```python
from build123d import *

# Parameters (mm, degrees)
SKETCH008_W  = 20
SKETCH008_H  = 20
PAD004_DEPTH = 3
PAD005_DEPTH = 3
SKETCH014_W  = 3
SKETCH014_H  = 3
PAD010_DEPTH = 1.5
SKETCH015_W  = 3
SKETCH015_H  = 3
PAD011_DEPTH = 1.5


with BuildPart() as part:
    # Sketch008 → Pad004 (new body)
    with BuildSketch(Plane.XZ):
        with BuildLine():
            Line((-68, -38.5), (3, -38.5))
            Line((3, -3), (3, -38.5))
            Line((0, -3), (3, -3))
            ThreePointArc((0, 3), (-6.5, 0), (0, -3))
            Line((0, 3), (3, 3))
            Line((3, 3), (3, 38.5))
            Line((3, 38.5), (-68, 38.5))
            Line((-68, 38.5), (-68, -38.5))
        make_face()
        with BuildLine():
            ThreePointArc((-12.5, 15), (-15, 17.5), (-17.5, 15))
            Line((-17.5, 15), (-17.5, -15))
            ThreePointArc((-17.5, -15), (-15, -17.5), (-12.5, -15))
            Line((-12.5, 15), (-12.5, -15))
        make_face(mode=Mode.SUBTRACT)
        with BuildLine():
            ThreePointArc((-47.5, 15), (-50, 17.5), (-52.5, 15))
            Line((-52.5, 15), (-52.5, -15))
            ThreePointArc((-52.5, -15), (-50, -17.5), (-47.5, -15))
            Line((-47.5, 15), (-47.5, -15))
        make_face(mode=Mode.SUBTRACT)
        with Locations((-32.5, 0)):
            Rectangle(SKETCH008_W, SKETCH008_H, mode=Mode.SUBTRACT)
    extrude(amount=PAD004_DEPTH)

    # Sketch009 → Pad005 (join)
    with BuildSketch(Plane.XY.offset(31)):
        Polygon((-5, 0), (-5, 4), (-4, 5.5), (-5, 7), (-7, 7), (-7, 0), align=None)
        Polygon((-60, 0), (-60, 4), (-61, 5.5), (-60, 7), (-58, 7), (-58, 0), align=None)
    pad005 = extrude(amount=-PAD005_DEPTH)

    # Mirrored001: Pad005 across XY
    add(pad005.mirror(Plane.XY))

    # Sketch014 → Pad010 (join, symmetric)
    with BuildSketch(Plane.XY.offset(-6)):
        with Locations((-1.5, 1.5)):
            Rectangle(SKETCH014_W, SKETCH014_H)
        with Locations((-63.5, 1.5)):
            Rectangle(SKETCH014_W, SKETCH014_H)
    extrude(amount=PAD010_DEPTH, both=True)

    # Sketch015 → Pad011 (join, symmetric)
    with BuildSketch(Plane.YZ.offset(-33)):
        with Locations((1.5, -34)):
            Rectangle(SKETCH015_W, SKETCH015_H)
        with Locations((1.5, 34)):
            Rectangle(SKETCH015_W, SKETCH015_H)
    extrude(amount=PAD011_DEPTH, both=True)


with BuildPart() as part_1:
    # Body003 placement: moved
    add(part.part.moved(Location((0, -55, 0))))


solid = part_1.part
```
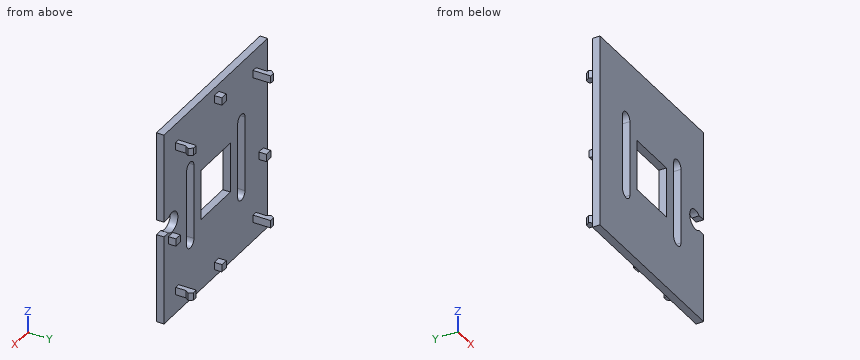
Verification items for the finished model (mm, model axes). Give positions to 0.01 mm unless a question says otherwise; leave off trailing zeros. Order: outer loops, then holes, each group sorted by start corner. A loop starts at its lowest first (then second) coordinate and runs counter-clockwise, first axis right, second up. Notation, with made-up numbers: (31, 64) - (40, 64) arc R23 cw to (40, 82) - close; hole circle Ø6 at (89, 78.25). An arc over 180 degrees is marked (long way). Answer as CSV lines item,"result". Start each with the question number.
Item 1: Gauge pin test, flat ends, axial feed: pin 1 (5 mm diameter, centred on x = -12.5, z = 13.5, fed in from +Y); pin 2 (0.9 mm diameter, centred on y = -53.5, z = -6, fed in from -X); pin 3 (2.5 mm diameter, centred on y = -50.5, z = -29.5, fed in from -X). Record the tip position at first contact, or that the pin passes through.
Item 2: Section check B-B, the plane y = -53.5. State how many separate pieces and enclosed holes the cut face has, plus the area to 3 significant figures.
Item 3: Section check C-C, the plane z = 6. Record the boundary of the cut face in (x, y).
Item 4: Section check D-D, the plane z = -13.5. Record the boundary of the cut face in (x, y), plus the area to 3 significant figures.
Item 5: Material ranges on L1, parallel to X at y = -56.75, z = 0; L2, parallel to X at y = -51, z = 30; L3, parallel to Z at x = -39, y = -57.5, recorded low to high.
Item 6: Section check A-A, the plane x = -15. Record the boundary of the cut face in (y, z), plus the area to 3 significant figures.
Filled in:
1,pin 1,"y = -55"
1,pin 2,"x = -65"
1,pin 3,"x = -61"
2,separate pieces,"8"
2,enclosed holes,"0"
2,area,"60.0 mm^2"
3,outline,"(-68, -58) - (-52.5, -58) - (-52.5, -55) - (-68, -55) - close; (-47.5, -58) - (-42.5, -58) - (-42.5, -55) - (-47.5, -55) - close; (-22.5, -58) - (-17.5, -58) - (-17.5, -55) - (-22.5, -55) - close; (-12.5, -58) - (3, -58) - (3, -55) - (-12.5, -55) - close"
4,outline,"(-68, -58) - (-52.5, -58) - (-52.5, -55) - (-68, -55) - close; (-47.5, -58) - (-17.5, -58) - (-17.5, -55) - (-47.5, -55) - close; (-12.5, -58) - (3, -58) - (3, -55) - (-12.5, -55) - close"
4,area,"183 mm^2"
5,L1,"-68 to -52.5, -47.5 to -42.5, -22.5 to -17.5, -12.5 to -6.5"
5,L2,"-60 to -58, -7 to -5"
5,L3,"-38.5 to -10, 10 to 38.5"
6,outline,"(-58, -38.5) - (-55, -38.5) - (-55, -17.5) - (-58, -17.5) - close; (-58, 17.5) - (-55, 17.5) - (-55, 38.5) - (-58, 38.5) - close"
6,area,"126 mm^2"
